Here's how the part is built. I have some questions about the finished solid (model axes, mm). A direction names the side the tool comes from. Round coordinates to 2 decimals unless told otherwise and drop trailing zeros. Write each loop counter-clockwise with the first axis right and the second up, starting at its lowest first coordinate (ties: lowest second). Pieces come first, ordered by that corner, then holes. Notation, with made-up numbers: (-23.75, 12.5) - (5.25, 12.5) arc R28 ccw to (5.25, 42.5) - close; hole circle Ø11 at (6.25, 85.5). An arc over 180 degrees is marked (long way). Write item = value, one per line. Start each with the question number.
Item 1: Which directions (+Z, -Z, +X, -X, +Y, -Y) give clear straight access to the entire face, cutting with the end or side of a thin tool? Please do faces 3 (the face through (0.52, 29.843, 5.683)), 4 (the face through (-25.7, -24, 1.6)), 5 (the face through (-22.809, 18.475, 1.627)).
Item 2: For P1, Ø5.5, axis at x = 27.5, y = -20.5, coming from the -Z side; P2, Ø4, axis at x = -25, z = 3.5, coming from the +Y side; P3, Ø2.5, axis at y = 0.5, z = 1, coming from the -X side, each with a flat end and sliding along its axis, tell me the tip position at first contact or that it passes through.
Item 3: If we section it at A-A (x = 0): Please give me the cut outline in (y, z), and give its area (3 significant figures).
Item 4: If I drill on line 1 along Y through (x, z) = (0, 4.9); line 2 along X through (y, z) = (1.5, 7.5); line 3 along X through (y, z) = (-2, 4.5), over which ranges is the centre line in solid material (lowest first)? Write a range as [from, to].
Item 5: If we section it at C-C (z = 7): Give the number of separate pieces and of enclosed holes in the cut face, and give its area (3 significant figures).
Item 6: Thinking about a two-plate mould opening in X: for faces 1 (the face through (28.538, -22.996, 5.683)), 2 (the face through (-31, -15, 4)), which applies, pulls with the +X half, pulls with the -X half, needs draft (parallel to the pull), parting line crosses it, or undercut?
Item 7: If we section it at B-B (y = -9.5): Please give me the cut outline in (x, z).
```python
from build123d import *

# Parameters (mm, degrees)
EXTRUDE_1_DEPTH          = 8
HOLE_WIZARD_M4_1_D       = 4.8
PATTERN_CIRCULAR_1_COUNT = 8
CHAMFER_1_SIZE           = 1
CUT_EXTRUDE_2_DEPTH      = 3.3
PATTERN_CIRCULAR_3_COUNT = 8
SKETCH_7_R               = 21
CUT_EXTRUDE_4_DEPTH      = 7
SKETCH_8_R               = 20
CUT_EXTRUDE_5_DEPTH      = 45.395945761
HOLE_WIZARD_M4_2_D       = 4.5
CUT_EXTRUDE_6_DEPTH      = 3.3


with BuildPart() as part:
    # ｽｹｯﾁ1 → ﾎﾞｽ - 押し出し1 (new body)
    with BuildSketch(Plane.XY):
        with BuildLine():
            Line((31, -31), (-31, -31))
            Line((-31, -31), (-31, 0))
            ThreePointArc((-31, 0), (0, 31), (31, 0))
            Line((31, 0), (31, -31))
        make_face()
    extrude(amount=EXTRUDE_1_DEPTH)

    # M4 すきま穴1 (through all)
    with Locations(Plane(origin=(0, 0, 0), x_dir=(1, 0, 0), z_dir=(0, 0, -1))):
        with Locations((0, -27.5)):
            hole_wizard_m4_1 = Hole(HOLE_WIZARD_M4_1_D / 2)

    # 円形ﾊﾟﾀｰﾝ1: M4 すきま穴1 ×8 about axis, 3 skipped
    pattern_circular_1_axis = Axis((0, 0, 0), (0, 0, -1))
    add([hole_wizard_m4_1.rotate(pattern_circular_1_axis, i * 360 / PATTERN_CIRCULAR_1_COUNT) for i in range(1, PATTERN_CIRCULAR_1_COUNT) if i not in (3, 4, 5)], mode=Mode.SUBTRACT)

    # 面取り1
    chamfer_1_edges = [part.edges().sort_by_distance(p)[0] for p in [
        (31, -15.5, 0),
        (0, -31, 0),
        (-31, -15.5, 0),
        (0, 31, 0),
        (31, -31, 4),
        (-31, -31, 4),
    ]]
    chamfer(chamfer_1_edges, length=CHAMFER_1_SIZE)

    # ｽｹｯﾁ5 → ｶｯﾄ - 押し出し2 (cut)
    with BuildSketch(Plane(origin=(0, 0, 0), x_dir=(-1, 0, 0), z_dir=(0, 0, -1))):
        Polygon((2.020725942, 24), (4.041451884, 27.5), (2.020725942, 31), (-2.020725942, 31), (-4.041451884, 27.5), (-2.020725942, 24), align=None)
    cut_extrude_2 = extrude(amount=-CUT_EXTRUDE_2_DEPTH, mode=Mode.SUBTRACT)

    # 円形ﾊﾟﾀｰﾝ3: ｶｯﾄ - 押し出し2 ×8 about axis, 3 skipped
    pattern_circular_3_axis = Axis((0, 0, 0), (0, 0, -1))
    add([cut_extrude_2.rotate(pattern_circular_3_axis, i * 360 / PATTERN_CIRCULAR_3_COUNT) for i in range(1, PATTERN_CIRCULAR_3_COUNT) if i not in (3, 4, 5)], mode=Mode.SUBTRACT)

    # ｽｹｯﾁ7 → ｶｯﾄ - 押し出し4 (cut)
    with BuildSketch(Plane.XY.offset(8)):
        Circle(SKETCH_7_R)
    extrude(amount=-CUT_EXTRUDE_4_DEPTH, mode=Mode.SUBTRACT)

    # ｽｹｯﾁ8 → ｶｯﾄ - 押し出し5 (cut, through all)
    with BuildSketch(Plane.XY.offset(1)):
        Circle(SKETCH_8_R)
    extrude(amount=-CUT_EXTRUDE_5_DEPTH, mode=Mode.SUBTRACT)

    # M4 すきま穴2 (through all)
    with Locations(Plane(origin=(0, 0, 0), x_dir=(-1, 0, 0), z_dir=(0, 0, -1))):
        with Locations((-27.5, -21), (27.5, -21)):
            Hole(HOLE_WIZARD_M4_2_D / 2)

    # ｽｹｯﾁ11 → ｶｯﾄ - 押し出し6 (cut)
    with BuildSketch(Plane(origin=(0, 0, 0), x_dir=(-1, 0, 0), z_dir=(0, 0, -1))):
        Polygon((-24, -23.020725942), (-24, -18.979274058), (-27.5, -16.958548116), (-31, -18.979274058), (-31, -23.020725942), (-27.5, -25.041451884), align=None)
        Polygon((27.5, -25.041451884), (31, -23.020725942), (31, -18.979274058), (27.5, -16.958548116), (24, -18.979274058), (24, -23.020725942), align=None)
    extrude(amount=-CUT_EXTRUDE_6_DEPTH, mode=Mode.SUBTRACT)


solid = part.part
```
Reply:
q1.face_3 = +Z, -Z
q1.face_4 = -Z
q1.face_5 = -Z, +Y
q2.P1 = 3.3
q2.P2 = 20.78
q2.P3 = -24
q3.outline = (-31, 1) - (-30, 0) - (-20, 0) - (-20, 1) - (-21, 1) - (-21, 8) - (-31, 8) - close; (20, 0) - (24, 0) - (24, 3.3) - (25.1, 3.3) - (25.1, 8) - (21, 8) - (21, 1) - (20, 1) - close; (29.9, 3.3) - (31, 3.3) - (31, 8) - (29.9, 8) - close
q3.area = 116 mm2
q4.line_1 = [-31, -21], [21, 25.1], [29.9, 31]
q4.line_2 = [-30.96, -29.37], [-25.63, -20.95], [20.95, 25.63], [29.37, 30.96]
q4.line_3 = [-31, -28.83], [-26.17, -20.9], [20.9, 26.17], [28.83, 31]
q5.separate_pieces = 1
q5.enclosed_holes = 8
q5.area = 1,920 mm2
q6.face_1 = undercut
q6.face_2 = pulls with the -X half
q7.outline = (-31, 1) - (-30, 0) - (-17.6, 0) - (-17.6, 1) - (-18.73, 1) - (-18.73, 8) - (-31, 8) - close; (17.6, 0) - (30, 0) - (31, 1) - (31, 8) - (18.73, 8) - (18.73, 1) - (17.6, 1) - close
